from build123d import *

# Parameters (mm, degrees)
SALIENTE_EXTRUIR1_DEPTH      = 32
CORTAR_EXTRUIR1_DEPTH        = 27
CROQUIS3_R                   = 62.5
CORTAR_EXTRUIR2_DEPTH        = 29
CROQUIS4_R                   = 18
SALIENTE_EXTRUIR2_DEPTH      = 8
CROQUIS5_R                   = 49
CORTAR_EXTRUIR3_DEPTH        = 5
SALIENTE_EXTRUIR3_DEPTH      = 5
SALIENTE_EXTRUIR4_REACH      = 167.907
SALIENTE_EXTRUIR5_DEPTH      = 5
CROQUIS9_R                   = 1.7
CORTAR_EXTRUIR4_DEPTH        = 8
CORTAR_EXTRUIR5_DEPTH        = 1.5
MATRIZC1_COUNT               = 3
SALIENTE_EXTRUIR6_DEPTH      = 12
CROQUIS12_R                  = 1.7
CORTAR_EXTRUIR6_DEPTH        = 12
CORTAR_EXTRUIR7_DEPTH        = 1.5
CORTAR_EXTRUIR7_DEPTH_BACK   = 1.5
CROQUIS14_R                  = 1.7
CORTAR_EXTRUIR8_DEPTH        = 58
CORTAR_EXTRUIR8_DEPTH_BACK   = 58.5
CROQUIS15_R                  = 1.7
CORTAR_EXTRUIR9_DEPTH        = 11.5
CROQUIS16_R                  = 2.95
CORTAR_EXTRUIR10_DEPTH       = 2.9
REDONDEO1_R                  = 5
CROQUIS17_R                  = 4.2
CORTAR_EXTRUIR11_DEPTH       = 1.1
SALIENTE_EXTRUIR7_DEPTH      = 3
SALIENTE_EXTRUIR7_DEPTH_BACK = 3
CROQUIS19_R                  = 75
CORTAR_EXTRUIR12_DEPTH       = 35
CORTAR_EXTRUIR13_DEPTH       = 27


with BuildPart() as part:
    # Croquis1 → Saliente-Extruir1 (new body)
    with BuildSketch(Plane(origin=(0, 0, 0), x_dir=(1, 0, 0), z_dir=(0, 1, 0))):
        with BuildLine():
            ThreePointArc((51.23475383, 40), (0, 145), (-51.23475383, 40))
            ThreePointArc((-51.23475383, 40), (-37.46950766, 0), (-51.23475383, -40))
            ThreePointArc((-51.23475383, -40), (0, -145), (51.23475383, -40))
            ThreePointArc((51.23475383, -40), (37.46950766, 0), (51.23475383, 40))
        make_face()
    extrude(amount=SALIENTE_EXTRUIR1_DEPTH)

    # Croquis2 → Cortar-Extruir1 (cut)
    with BuildSketch(Plane(origin=(0, 32, 0), x_dir=(1, 0, 0), z_dir=(0, 1, 0))):
        with BuildLine():
            ThreePointArc((47.29361892, 43.076923077), (0, 140), (-47.29361892, 43.076923077))
            ThreePointArc((-47.29361892, 43.076923077), (-32.46950766, 0), (-47.29361892, -43.076923077))
            ThreePointArc((-47.29361892, -43.076923077), (0, -140), (47.29361892, -43.076923077))
            ThreePointArc((47.29361892, -43.076923077), (32.46950766, 0), (47.29361892, 43.076923077))
        make_face()
    extrude(amount=-CORTAR_EXTRUIR1_DEPTH, mode=Mode.SUBTRACT)

    # Croquis3 → Cortar-Extruir2 (cut)
    with BuildSketch(Plane(origin=(0, 32, 0), x_dir=(1, 0, 0), z_dir=(0, 1, 0))):
        with Locations(Location((0, -80, 0), (0, 0, 270))):
            Circle(CROQUIS3_R)
    extrude(amount=-CORTAR_EXTRUIR2_DEPTH, mode=Mode.SUBTRACT)

    # Croquis4 → Saliente-Extruir2 (add)
    with BuildSketch(Plane(origin=(0, 3, 0), x_dir=(1, 0, 0), z_dir=(0, 1, 0))):
        with Locations(Location((0, -80, 0), (0, 0, 270))):
            Circle(CROQUIS4_R)
    extrude(amount=SALIENTE_EXTRUIR2_DEPTH)

    # Croquis5 → Cortar-Extruir3 (cut)
    with BuildSketch(Plane.XZ):
        with Locations(Location((0, -80, 0), (0, 0, 270))):
            Circle(CROQUIS5_R)
    extrude(amount=-CORTAR_EXTRUIR3_DEPTH, mode=Mode.SUBTRACT)

    # Croquis6 → Saliente-Extruir3 (add)
    with BuildSketch(Plane(origin=(0, 5, 0), x_dir=(1, 0, 0), z_dir=(0, 1, 0))):
        with BuildLine():
            ThreePointArc((-33.685420375, 12.990355514), (0, 5), (33.685420375, 12.990355514))
            ThreePointArc((33.685420375, 12.990355514), (32.46950766, 0), (33.685420375, -12.990355514))
            ThreePointArc((33.685420375, -12.990355514), (0, -5), (-33.685420375, -12.990355514))
            ThreePointArc((-33.685420375, -12.990355514), (-32.46950766, 0), (-33.685420375, 12.990355514))
        make_face()
    extrude(amount=SALIENTE_EXTRUIR3_DEPTH)

    # Croquis7 → Saliente-Extruir4 (add, up to next)
    with BuildSketch(Plane(origin=(9, 0, 0), x_dir=(0, 0, -1), z_dir=(1, 0, 0)), mode=Mode.PRIVATE) as saliente_extruir4_sk1:
        Polygon((11, 8.038971661), (11, 5), (13.45, 5), (16, 8.038971661), align=None)
    saliente_extruir4_tool1 = extrude(saliente_extruir4_sk1.sketch, amount=SALIENTE_EXTRUIR4_REACH, mode=Mode.PRIVATE) - part.part
    # Croquis7 → Saliente-Extruir4 (add, up to next)
    with BuildSketch(Plane(origin=(9, 0, 0), x_dir=(0, 0, -1), z_dir=(1, 0, 0)), mode=Mode.PRIVATE) as saliente_extruir4_sk2:
        Polygon((23.7, 8.038971661), (28.7, 8.038971661), (28.7, 5), (26.25, 5), align=None)
    saliente_extruir4_tool2 = extrude(saliente_extruir4_sk2.sketch, amount=SALIENTE_EXTRUIR4_REACH, mode=Mode.PRIVATE) - part.part
    saliente_extruir4_1 = saliente_extruir4_tool1.solids().sort_by_distance((9, 6.69285, -12.935235))[0]
    add(saliente_extruir4_1)
    saliente_extruir4_2 = saliente_extruir4_tool2.solids().sort_by_distance((9, 6.69285, -26.764765))[0]
    add(saliente_extruir4_2)
    saliente_extruir4 = saliente_extruir4_1 + saliente_extruir4_2  # Saliente-Extruir4 as one shape, for the pattern or mirror that repeats it

    # Simetr_a1: Saliente-Extruir4 across plane
    add(saliente_extruir4.mirror(Plane(origin=(0, 0, 0), x_dir=(0, 0, 1), z_dir=(1, 0, 0))))

    # Croquis8 → Saliente-Extruir5 (add, symmetric)
    with BuildSketch(Plane(origin=(0, 0, 0), x_dir=(0, 0, -1), z_dir=(1, 0, 0))):
        Polygon((121, 13), (141, 13), (141, 5), (129, 5), (129, 7), (121, 7), align=None)
    saliente_extruir5 = extrude(amount=SALIENTE_EXTRUIR5_DEPTH, both=True)

    # Croquis9 → Cortar-Extruir4 (cut)
    with BuildSketch(Plane(origin=(0, 13, 0), x_dir=(1, 0, 0), z_dir=(0, 1, 0))):
        with Locations(Location((0, 125, 0), (0, 0, 270))):
            Circle(CROQUIS9_R)
    cortar_extruir4 = extrude(amount=-CORTAR_EXTRUIR4_DEPTH, mode=Mode.SUBTRACT)

    # Croquis10 → Cortar-Extruir5 (cut, symmetric)
    with BuildSketch(Plane(origin=(0, 10, 0), x_dir=(1, 0, 0), z_dir=(0, 1, 0))):
        Polygon((-2.901185103, 123.325), (-2.901185103, 116.675), (2.901185103, 116.675), (2.901185103, 123.325), (2.901185103, 126.675), (0, 128.35), (-2.901185103, 126.675), align=None)
    cortar_extruir5 = extrude(amount=CORTAR_EXTRUIR5_DEPTH, both=True, mode=Mode.SUBTRACT)

    # MatrizC1: Saliente-Extruir5, Cortar-Extruir4, Cortar-Extruir5 ×3 about axis
    matrizc1_axis = Axis((0, 0, -80), (0, 1, 0))
    add([saliente_extruir5.rotate(matrizc1_axis, i * 360 / MATRIZC1_COUNT) for i in range(1, MATRIZC1_COUNT)])
    add([cortar_extruir4.rotate(matrizc1_axis, i * 360 / MATRIZC1_COUNT) for i in range(1, MATRIZC1_COUNT)], mode=Mode.SUBTRACT)
    add([cortar_extruir5.rotate(matrizc1_axis, i * 360 / MATRIZC1_COUNT) for i in range(1, MATRIZC1_COUNT)], mode=Mode.SUBTRACT)

    # Croquis11 → Saliente-Extruir6 (add)
    with BuildSketch(Plane(origin=(0, 13, 0), x_dir=(1, 0, 0), z_dir=(0, 1, 0))):
        with BuildLine():
            Line((5, 130), (-5, 130))
            Line((-5, 130), (-5, 139.791303716))
            ThreePointArc((-5, 139.791303716), (0, 140), (5, 139.791303716))
            Line((5, 139.791303716), (5, 130))
        make_face()
    extrude(amount=SALIENTE_EXTRUIR6_DEPTH)

    # Croquis12 → Cortar-Extruir6 (cut)
    with BuildSketch(Plane(origin=(0, 25, 0), x_dir=(1, 0, 0), z_dir=(0, 1, 0))):
        with Locations(Location((0, 135, 0), (0, 0, 270))):
            Circle(CROQUIS12_R)
    extrude(amount=-CORTAR_EXTRUIR6_DEPTH, mode=Mode.SUBTRACT)

    # Croquis13 → Cortar-Extruir7 (cut, two sides)
    with BuildSketch(Plane(origin=(0, 20.5, 0), x_dir=(1, 0, 0), z_dir=(0, 1, 0))) as cortar_extruir7_sk:
        Polygon((-2.901185103, 133.325), (-2.901185103, 126.675), (2.901185103, 126.675), (2.901185103, 133.325), (2.901185103, 136.675), (0, 138.35), (-2.901185103, 136.675), align=None)
    extrude(amount=CORTAR_EXTRUIR7_DEPTH, mode=Mode.SUBTRACT)
    extrude(cortar_extruir7_sk.sketch, amount=-CORTAR_EXTRUIR7_DEPTH_BACK, mode=Mode.SUBTRACT)

    # Croquis14 → Cortar-Extruir8 (cut, two sides)
    with BuildSketch(Plane(origin=(0, 0, 0), x_dir=(0, 0, -1), z_dir=(1, 0, 0))) as cortar_extruir8_sk:
        with Locations(Location((19.85, 8.8, 0), (0, 0, 180))):
            Circle(CROQUIS14_R)
    extrude(amount=CORTAR_EXTRUIR8_DEPTH, mode=Mode.SUBTRACT)
    extrude(cortar_extruir8_sk.sketch, amount=-CORTAR_EXTRUIR8_DEPTH_BACK, mode=Mode.SUBTRACT)

    # Croquis15 → Cortar-Extruir9 (cut)
    with BuildSketch(Plane.XZ):
        with Locations(Location((-28.5, 6.5, 0), (0, 0, 270))):
            Circle(CROQUIS15_R)
        with Locations(Location((-28.5, -6.5, 0), (0, 0, 270))):
            Circle(CROQUIS15_R)
        with Locations(Location((28.5, 6.5, 0), (0, 0, 270))):
            Circle(CROQUIS15_R)
        with Locations(Location((28.5, -6.5, 0), (0, 0, 270))):
            Circle(CROQUIS15_R)
    extrude(amount=-CORTAR_EXTRUIR9_DEPTH, mode=Mode.SUBTRACT)

    # Croquis16 → Cortar-Extruir10 (cut)
    with BuildSketch(Plane.XZ):
        with Locations(Location((-28.5, 6.5, 0), (0, 0, 270))):
            Circle(CROQUIS16_R)
        with Locations(Location((-28.5, -6.5, 0), (0, 0, 270))):
            Circle(CROQUIS16_R)
        with Locations(Location((28.5, 6.5, 0), (0, 0, 270))):
            Circle(CROQUIS16_R)
        with Locations(Location((28.5, -6.5, 0), (0, 0, 270))):
            Circle(CROQUIS16_R)
    extrude(amount=-CORTAR_EXTRUIR10_DEPTH, mode=Mode.SUBTRACT)

    # Redondeo1
    redondeo1_edges = [part.edges().sort_by_distance(p)[0] for p in [
        (0, 0, 145),
        (-37.46950766, 0, 0),
        (0, 0, -145),
        (37.46950766, 0, 0),
    ]]
    fillet(redondeo1_edges, radius=REDONDEO1_R)

    # Croquis17 → Cortar-Extruir11 (cut)
    with BuildSketch(Plane.XZ):
        with Locations(Location((0, 0, 0), (0, 0, 270))):
            Circle(CROQUIS17_R)
        with Locations(Location((0, -134.5, 0), (0, 0, 270))):
            Circle(CROQUIS17_R)
    extrude(amount=-CORTAR_EXTRUIR11_DEPTH, mode=Mode.SUBTRACT)

    # Croquis18 → Saliente-Extruir7 (add, two sides)
    with BuildSketch(Plane.XY) as saliente_extruir7_sk:
        Polygon((-35, 27), (-35, 17), (-25, 27), align=None)
        Polygon((25, 27), (35, 27), (35, 17), align=None)
    extrude(amount=SALIENTE_EXTRUIR7_DEPTH)
    extrude(saliente_extruir7_sk.sketch, amount=-SALIENTE_EXTRUIR7_DEPTH_BACK)

    # Croquis19 → Cortar-Extruir12 (cut)
    with BuildSketch(Plane.XZ):
        with Locations((0, 80)):
            Circle(CROQUIS19_R)
    extrude(amount=-CORTAR_EXTRUIR12_DEPTH, mode=Mode.SUBTRACT)

    # Croquis20 → Cortar-Extruir13 (cut)
    with BuildSketch(Plane(origin=(0, 32, 0), x_dir=(1, 0, 0), z_dir=(0, 1, 0))):
        with BuildLine():
            Line((-50, 24.098300563), (-50, -24.098300563))
            ThreePointArc((-50, -24.098300563), (0, -5), (50, -24.098300563))
            Line((50, -24.098300563), (50, 24.098300563))
            ThreePointArc((50, 24.098300563), (0, 5), (-50, 24.098300563))
        make_face()
    extrude(amount=-CORTAR_EXTRUIR13_DEPTH, mode=Mode.SUBTRACT)


solid = part.part
Can you work these out from the model? Positions are in its coordinate system, mm. A direction names the side the tool comes from. Round coordinates to 2 decimals unless told otherwise and drop trailing zeros. Write each question's results on one line, items separated by ' | '. Start each with the question number.
1) Which directions (+Z, -Z, +X, -X, +Y, -Y) give clear straight access to the entire face, cutting with the end or side of a thin tool? Please do faces 4 (the flat face through (0, 18, -130)), 5 (the flat face through (-35.54, 11.96, -59.56)), 6 (the flat face through (0, 13, -135)), 7 (the cylindrical face through (1.262, 0.542, -4.006)), 8 (the flat face through (42.4, 5.99, -55.44)).
2) Please list where these lines run through material, in increasing order: line 1 (Z direction, x = -28, y = 1); line 2 (X direction, y = 2.1, z = -6.5); line 3 (Y direction, x = 28, z = -29).
3) For pin 1 Ø4.5 at (x, z) = (-28, 5.5) entering from -Y; pin 2 Ø5 at (x, y) = (49, 6) entering from -Z; pin 3 Ø10 at (y, z) = (27, -28) entering from +X; pin 4 Ø3 at (x, y) = (2, 11) entering from +Z, each with a flat end and sliding along its axis, tell me the tip position at first contact or that it passes through.
4) We'd pull the mould along Z, two halves only. Please class faces 1 (the cylindrical face through (1.433, 16.042, -134.086)), 2 (the flat face through (-1, 19, -133)), 3 (the cylindrical face through (-36.73, 18.69, -14.61)): released by +Z, released by -Z, zero draft, split by the parting line, or undercut.
Here are the results:
1) face 4: +Z, +Y | face 5: +Y, -Y | face 6: +Y | face 7: -Y | face 8: none
2) line 1: z = -136.44 to -120.21, -39.79 to -9.41, -3.59 to 3.59, 9.41 to 10.42 | line 2: x = -36.86 to -31.45, -25.55 to 25.55, 31.45 to 36.86 | line 3: y = 0 to 5
3) pin 1: stops at y = 0 | pin 2: stops at z = -125.42 | pin 3: stops at x = 46.47 | pin 4: stops at z = -121
4) face 1: undercut | face 2: zero draft | face 3: released by +Z
